Design review of the part built by this model. Coordinates are the model's own, in mm. Coordinates: 2 decimals unless noted, no trailing zeros. Order: outer loops, then holes, each group sorted by start corner. A loop starts at its lowest first (then second) coordinate and runs counter-clockwise, first axis right, second up. Notation, with made-up numbers: (25.5, 20) -> (61.5, 20) arc R5 ccw to (61.5, 27) -> close; hole circle Ø2 at (46, 57). An arc over 180 degrees is marked (long way). Write item = value, one per line.
```python
from build123d import *

# Parameters (mm, degrees)
F1_DEPTH   = 12
F3_D       = 20
F4_C1_SIZE = 1
F4_C2_SIZE = 1
F4_C3_SIZE = 1
F4_C4_SIZE = 1
F4_C5_SIZE = 1
F4_C6_SIZE = 1
F4_C7_SIZE = 1
F4_C8_SIZE = 0.9999
F5_C1_SIZE = 1
F5_C2_SIZE = 1
F5_C3_SIZE = 1
F5_C4_SIZE = 1
F5_C5_SIZE = 1
F5_C6_SIZE = 1
F5_C7_SIZE = 1
F5_C8_SIZE = 0.9999


# Not quite as in the source:
# - a fillet or chamfer is up to 0.001 mm smaller than in the source, because OpenCascade refuses the exact size


with BuildPart() as f1:
    # F0 (on Front) → F1 (new body)
    with BuildSketch(Plane.XZ):
        with BuildLine():
            ThreePointArc((-70.6781876117, 0), (0, -56.3108485805), (70.6781876117, 0))
            ThreePointArc((70.6781876117, 0), (40.1621081353, 14.7607018174), (25, 45.079341326))
            ThreePointArc((25, 45.079341326), (0, 20.079341326), (-25, 45.079341326))
            ThreePointArc((-25, 45.079341326), (-40.2089612492, 14.808177341), (-70.6781876117, 0))
        make_face()
        with BuildLine():
            ThreePointArc((-25, 45.079341326), (0, 20.079341326), (25, 45.079341326))
            Line((25, 45.079341326), (-25, 45.079341326))
        make_face()
        with BuildLine():
            Line((-25, 45.079341326), (25, 45.079341326))
            ThreePointArc((25, 45.079341326), (0, 70.079341326), (-25, 45.079341326))
        make_face()
    extrude(amount=F1_DEPTH)

    # F3 (through all)
    with Locations(Plane(origin=(0, 0, 0), x_dir=(-1, 0, 0), z_dir=(0, 1, 0))):
        with Locations((-40.0044433773, -15.3863234445), (0, -35.2486670017), (39.1651876271, -16.7850796133), (0, 47.8374771774)):
            Hole(F3_D / 2)

    # F4: chamfer of 1 on 8 edges, made by hand

    # F4_c1
    f4_c1_edges = [f1.edges().sort_by_distance(p)[0] for p in [
        (40.1621081353, 0, 14.7607018174),
    ]]
    chamfer(f4_c1_edges, length=F4_C1_SIZE)

    # F4_c2
    f4_c2_edges = [f1.edges().sort_by_distance(p)[0] for p in [
        (-0.5029833863, 0, -56.3091040511),
    ]]
    chamfer(f4_c2_edges, length=F4_C2_SIZE)

    # F4_c3
    f4_c3_edges = [f1.edges().sort_by_distance(p)[0] for p in [
        (-39.8532973479, 0, 15.1625303947),
    ]]
    chamfer(f4_c3_edges, length=F4_C3_SIZE)

    # F4_c4
    f4_c4_edges = [f1.edges().sort_by_distance(p)[0] for p in [
        (10, 0, -35.2486670017),
    ]]
    chamfer(f4_c4_edges, length=F4_C4_SIZE)

    # F4_c5
    f4_c5_edges = [f1.edges().sort_by_distance(p)[0] for p in [
        (-29.1651876271, 0, -16.7850796133),
    ]]
    chamfer(f4_c5_edges, length=F4_C5_SIZE)

    # F4_c6
    f4_c6_edges = [f1.edges().sort_by_distance(p)[0] for p in [
        (50.0044433773, 0, -15.3863234445),
    ]]
    chamfer(f4_c6_edges, length=F4_C6_SIZE)

    # F4_c7
    f4_c7_edges = [f1.edges().sort_by_distance(p)[0] for p in [
        (10, 0, 47.8374771774),
    ]]
    chamfer(f4_c7_edges, length=F4_C7_SIZE)

    # F4_c8 (size 1 in the source; OpenCascade refuses exactly that, so slightly less here)
    f4_c8_edges = [f1.edges().sort_by_distance(p)[0] for p in [
        (0, 0, 70.079341326),
    ]]
    chamfer(f4_c8_edges, length=F4_C8_SIZE)

    # F5: chamfer of 1 on 8 edges, made by hand

    # F5_c1
    f5_c1_edges = [f1.edges().sort_by_distance(p)[0] for p in [
        (40.1621081353, -12, 14.7607018174),
    ]]
    chamfer(f5_c1_edges, length=F5_C1_SIZE)

    # F5_c2
    f5_c2_edges = [f1.edges().sort_by_distance(p)[0] for p in [
        (-0.5029833863, -12, -56.3091040511),
    ]]
    chamfer(f5_c2_edges, length=F5_C2_SIZE)

    # F5_c3
    f5_c3_edges = [f1.edges().sort_by_distance(p)[0] for p in [
        (-39.8532973479, -12, 15.1625303947),
    ]]
    chamfer(f5_c3_edges, length=F5_C3_SIZE)

    # F5_c4
    f5_c4_edges = [f1.edges().sort_by_distance(p)[0] for p in [
        (10, -12, 47.8374771774),
    ]]
    chamfer(f5_c4_edges, length=F5_C4_SIZE)

    # F5_c5
    f5_c5_edges = [f1.edges().sort_by_distance(p)[0] for p in [
        (50.0044433773, -12, -15.3863234445),
    ]]
    chamfer(f5_c5_edges, length=F5_C5_SIZE)

    # F5_c6
    f5_c6_edges = [f1.edges().sort_by_distance(p)[0] for p in [
        (-29.1651876271, -12, -16.7850796133),
    ]]
    chamfer(f5_c6_edges, length=F5_C6_SIZE)

    # F5_c7
    f5_c7_edges = [f1.edges().sort_by_distance(p)[0] for p in [
        (10, -12, -35.2486670017),
    ]]
    chamfer(f5_c7_edges, length=F5_C7_SIZE)

    # F5_c8 (size 1 in the source; OpenCascade refuses exactly that, so slightly less here)
    f5_c8_edges = [f1.edges().sort_by_distance(p)[0] for p in [
        (0, -12, 70.079341326),
    ]]
    chamfer(f5_c8_edges, length=F5_C8_SIZE)


solid = f1.part
```
(1) For L1, parallel to X at y = -4, z = -13; L2, parallel to X at y = -6.5, z = -7.5; L3, parallel to Z at x = -7.5, y = -9, list the stretches that pass through material, from the lowest coordinate up.
Report:
L1 = -66.37 to -48.42, -29.91 to 30.29, 49.72 to 66.37
L2 = -68.53 to -42.88, -35.45 to 33.86, 46.15 to 68.53
L3 = -55.92 to -41.86, -28.63 to 41.22, 54.45 to 68.93
(2) The part is to be moulded in two halves that separate along X. For faces 1 (the cylindrical face through (0.55, -5.93, 70.073)), 2 (the cylindrical face through (-29.627, -6.07, -13.781)), 3 (the conical face through (40.363, -11.174, 14.321)), 4 (the flat face through (-1, -12, -6)), say which applies: released by +X, released by -X, zero draft, split by the parting line, or undercut.
Report:
face_1 = split by the parting line
face_2 = undercut
face_3 = released by +X
face_4 = zero draft
(3) Insertion check: pin 1 (1.5 mm diameter, centred on x = 28.5, y = -6.5, fed in from -Z); pin 2 (1 mm diameter, centred on x = -3, y = -8, fed in from +Z); pin 3 (4 mm diameter, centred on y = -5.5, z = 18, fed in from +X). Each pin has a flat end and moves straight along its axis. Give the tip position at first contact, or say it passes through.
Report:
pin_1 = -50.79
pin_2 = 69.95
pin_3 = 38.95
(4) We need section A-A (x = 0). Write out the cut boundary in (y, z).
Report:
outline = (-12, -55.31) -> (-11, -56.31) -> (-1, -56.31) -> (0, -55.31) -> (0, -46.25) -> (-1, -45.25) -> (-11, -45.25) -> (-12, -46.25) -> close; (-12, -24.25) -> (-11, -25.25) -> (-1, -25.25) -> (0, -24.25) -> (0, 36.84) -> (-1, 37.84) -> (-11, 37.84) -> (-12, 36.84) -> close; (-12, 58.84) -> (-11, 57.84) -> (-1, 57.84) -> (0, 58.84) -> (0, 69.08) -> (-1, 70.08) -> (-11, 70.08) -> (-12, 69.08) -> close
(5) We need section B-B (y = -8.25). Write out the cut boundary in (x, z), and give its area (3 significant figures).
Report:
outline = (-70.68, 0) arc R72.51 ccw to (70.68, 0) arc R52.57 cw to (25, 45.08) arc R25 ccw to (-25, 45.08) arc R52.83 cw to start; hole circle Ø20 at (-39.17, -16.79); hole circle Ø20 at (0, -35.25); hole circle Ø20 at (0, 47.84); hole circle Ø20 at (40, -15.39)
area = 9,010 mm²
